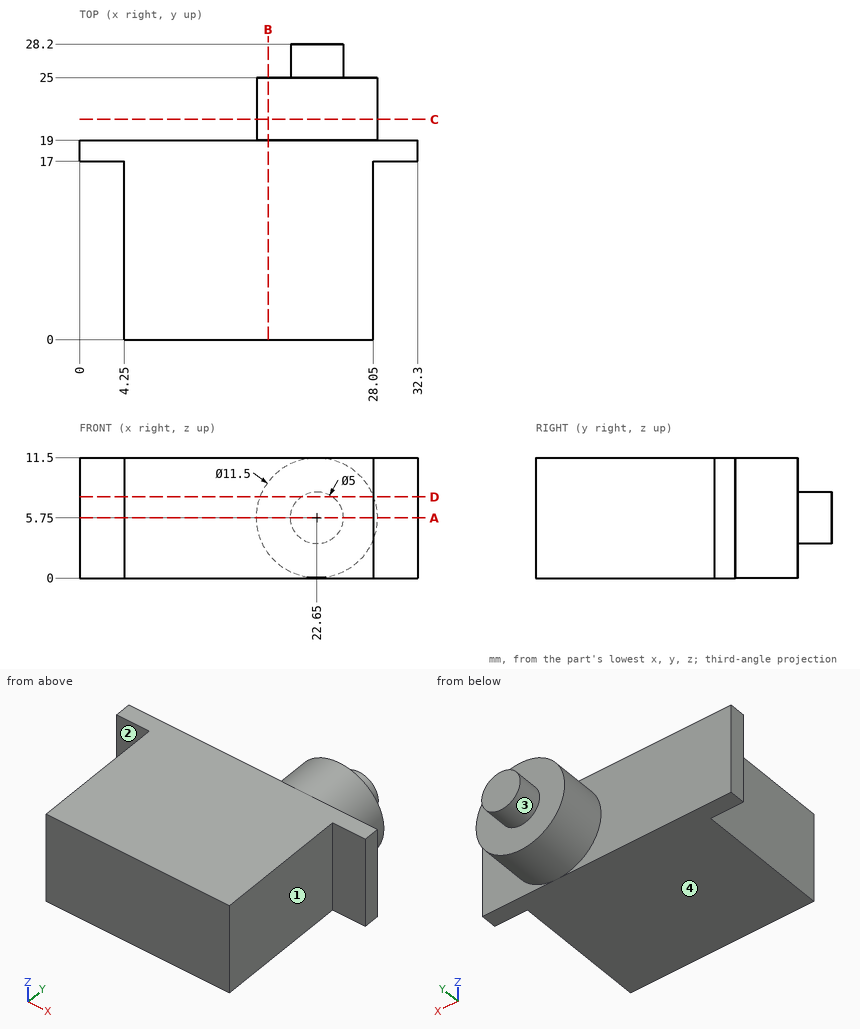
The drawing under review shows one solid part. Ordinate dimensions are in mm from its lowest x, y, z. A direction names the side the tool comes from. Coordinates: 2 decimals unless noted, no trailing zeros. Write each loop counter-clockwise with the first axis right and the second up, starting at its lowest first coordinate (ties: lowest second). Pieces come first, ordered by that corner, then holes. Notation, with made-up numbers: M 63.5,64.5 L 109.5,64.5 A7 cw 109.5,70.5 Z; hole C 52,-34 d4. An arc over 180 degrees is marked long. Put each result on its own line as item: value.
1) Add section A-A on z = 5.75. Give the boundary of the cut face in (x, y).
Computed:
outline: M 0,17 L 4.25,17 L 4.25,0 L 28.05,0 L 28.05,17 L 32.3,17 L 32.3,19 L 28.4,19 L 28.4,25 L 25.15,25 L 25.15,28.2 L 20.15,28.2 L 20.15,25 L 16.9,25 L 16.9,19 L 0,19 Z
2) Add section C-C on y = 21. Give the boundary of the cut face in (x, z).
Computed:
outline: C 22.65,5.75 d11.5
3) For the marked faces 1, 2, 3 and 4, list the 3-axis set-ups (+Z, -Z, +X, -X, +Y, -Y) from which the entire face can be reached by the end or side of a thin tool; tool diameter is ignored.
Computed:
face 1: +Z, -Z, +X, -Y
face 2: +Z, -Z, -X, -Y
face 3: +Y
face 4: -Z, +X, -X, +Y, -Y
4) Add section D-D on z = 7.75. Give the boundary of the cut face in (x, y).
Computed:
outline: M 0,17 L 4.25,17 L 4.25,0 L 28.05,0 L 28.05,17 L 32.3,17 L 32.3,19 L 28.04,19 L 28.04,25 L 24.15,25 L 24.15,28.2 L 21.15,28.2 L 21.15,25 L 17.26,25 L 17.26,19 L 0,19 Z
5) Clearance check with flat-ended pins moving along their axes: pin 1 Ø3.5 at (x, z) = (30.5, 7) entering from -Y; pin 2 Ø3 at (x, z) = (7, 2.5) entering from +Y; pin 3 Ø5 at (y, z) = (7.5, 5.5) entering from +X; pin 4 Ø3 at (x, z) = (26, 5) entering from +Y. State where each tip first meets the part, or that it passes through.
Computed:
pin 1: stops at y = 17
pin 2: stops at y = 19
pin 3: stops at x = 28.05
pin 4: stops at y = 28.2
6) Wall thickness on probe 1 along Y at (x, z) = (7.5, 8); probe 2 along X at (y, z) = (11, 5.25); probe 3 along Y at (x, z) = (29.5, 7.5): over which ranges is each line inside the solid? List them lowest first. Write a range as [from, to].
Computed:
probe 1: y = [0, 19]
probe 2: x = [4.25, 28.05]
probe 3: y = [17, 19]
7) Add section B-B on x = 18. Give the boundary of the cut face in (y, z).
Computed:
outline: M 0,0 L 19,0 L 19,2.37 L 25,2.37 L 25,9.13 L 19,9.13 L 19,11.5 L 0,11.5 Z
